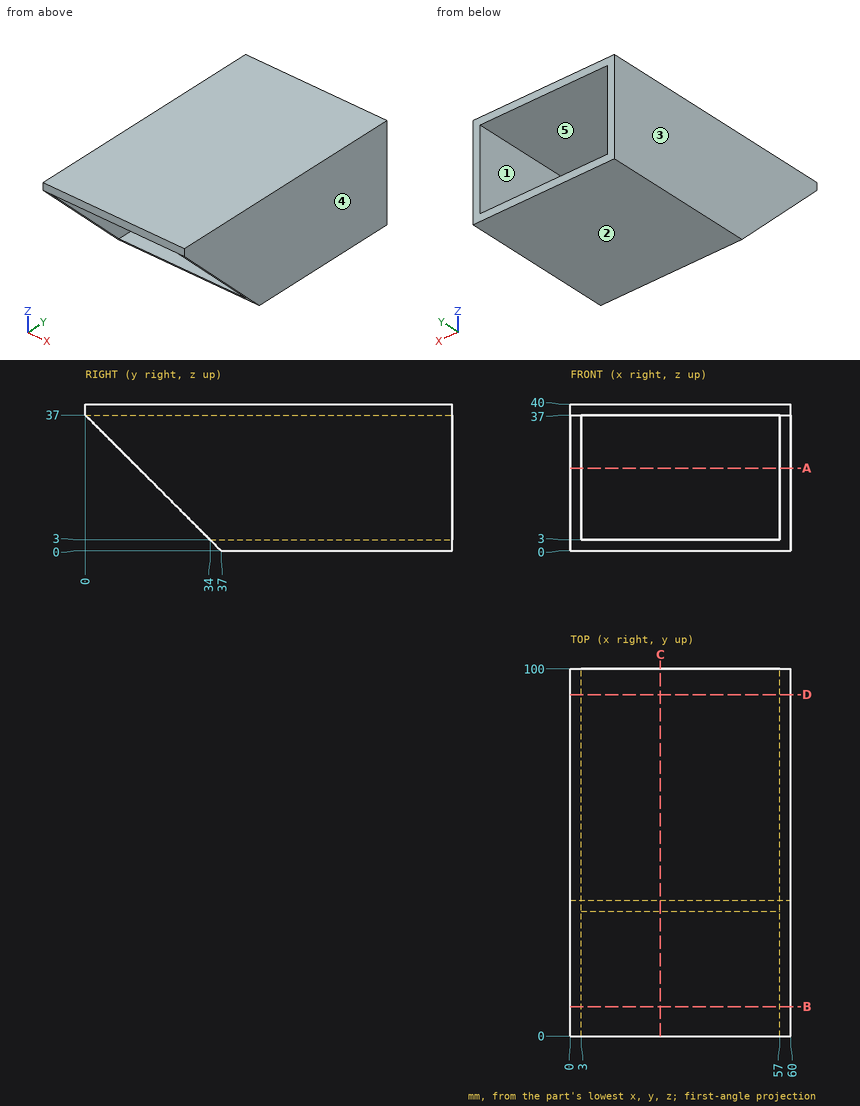
Part print with two shaded views. Sizes in mm from the minimum x, y, z corner. A direction names the side the tool comes from. Give positions to 0.01 mm unless a question says otherwise; leave off trailing zeros. Order: outer loops, then holes, each group sorted by start corner. A loop starts at its lowest first (then second) coordinate and runs counter-clockwise, first axis right, second up. Notation, with made-up numbers: M -19,88.25 L 39,88.25 A12 cw 39,102.25 Z; hole C -15,-13.5 d6. An arc over 180 degrees is marked long. Put each result on its own line as item: value.
Item 1: Cut at A-A on z = 22.5. Write the cut outline in (x, y), then the cut area to 3 significant figures.
Results are:
outline: M 0,14.5 L 3,14.5 L 3,100 L 0,100 Z; M 57,14.5 L 60,14.5 L 60,100 L 57,100 Z
area: 513 mm2
Item 2: Cut at D-D on y = 93. Write the cut outline in (x, z).
Results are:
outline: M 0,0 L 60,0 L 60,40 L 0,40 Z; hole M 3,3 L 57,3 L 57,37 L 3,37 Z
Item 3: Which spindle directions (+Z, -Z, +X, -X, +Y, -Y) get a long thin tool onto all of the face, cutting with end or side? Do the marked faces 4 and 5. Say none if no direction does.
Results are:
face 4: +Z, -Z, +X, +Y, -Y
face 5: +Y, -Y
Item 4: Pull direction X, two halves, no side cores. Call the marked faces 1, 2 and 3: +X half, -X half, draft (parallel to the pull), parting line (faces both ways), or undercut.
Results are:
face 1: undercut
face 2: draft
face 3: -X half
Item 5: Wall check: probe 1 along Z at (x, y) = (16.5, 43); probe 2 along X at (y, z) = (81, 10.5); probe 3 along Z at (x, y) = (19, 17.5). Give the ranges that are in metal, low to high.
Results are:
probe 1: 0 to 3, 37 to 40
probe 2: 0 to 3, 57 to 60
probe 3: 37 to 40
Item 6: Cut at C-C on x = 24.5. Write the cut outline in (y, z).
Results are:
outline: M 0,37 L 100,37 L 100,40 L 0,40 Z; M 34,3 L 37,0 L 100,0 L 100,3 Z
Item 7: Drop flat-ended pins along their axis: pin 1 Ø3 at (y, z) = (64, 4.5) entering from -X; pin 2 Ø10 at (x, y) = (47.5, 22) entering from -Z. Give the stop position or say it passes through.
Results are:
pin 1: x = 0
pin 2: z = 37
Item 8: Cut at B-B on y = 8. Write the cut outline in (x, z), then the cut area to 3 significant figures.
Results are:
outline: M 0,29 L 3,29 L 3,37 L 57,37 L 57,29 L 60,29 L 60,40 L 0,40 Z
area: 228 mm2
